Build history of the part. All positions in model axes, mm. Coordinates: 2 decimals unless noted, no trailing zeros. Order: outer loops, then holes, each group sorted by start corner. A loop starts at its lowest first (then second) coordinate and runs counter-clockwise, first axis right, second up. Notation, with made-up numbers: (26, 28) -> (44, 28) arc R25 cw to (44, 41) -> close; hole circle Ø9 at (28.5, 34). An arc over 180 degrees is marked (long way). Write each question's results on one line, items separated by ' | '.
from build123d import *

# Parameters (mm, degrees)
SKETCH1_R           = 2
BOSS_EXTRUDE1_DEPTH = 5.1


with BuildPart() as part:
    # Sketch1 → Boss-Extrude1 (new body)
    with BuildSketch(Plane.XY):
        with BuildLine():
            Line((-42.484250182, 62.101563959), (-42.484250182, 52.101563959))
            Line((-42.484250182, 52.101563959), (-57.610510686, 52.101563959))
            Line((-57.610510686, 52.101563959), (-57.610510686, 42.101563959))
            Line((-57.610510686, 42.101563959), (-2.484250182, -7.898436041))
            Line((-2.484250182, -7.898436041), (7.515749818, -7.898436041))
            Line((7.515749818, -7.898436041), (7.515749818, -17.898436041))
            Line((7.515749818, -17.898436041), (57.515749818, -17.898436041))
            Line((57.515749818, -17.898436041), (57.515749818, -7.898436041))
            Line((57.515749818, -7.898436041), (67.599923488, -7.898436041))
            Line((67.599923488, -7.898436041), (67.599923488, 2.101563959))
            Line((67.599923488, 2.101563959), (4.022842983, 38.364289155))
            ThreePointArc((4.022842983, 38.364289155), (3.080536426, 40.614131219), (5.013739676, 42.101563959))
            Line((5.013739676, 42.101563959), (22.642010323, 42.101563959))
            Line((22.642010323, 42.101563959), (22.642010323, 52.101563959))
            Line((22.642010323, 52.101563959), (7.515749818, 52.101563959))
            Line((7.515749818, 52.101563959), (7.515749818, 62.101563959))
            Line((7.515749818, 62.101563959), (-42.484250182, 62.101563959))
        make_face()
        with Locations((-32.484250182, 59.201563959)):
            Circle(SKETCH1_R, mode=Mode.SUBTRACT)
        with Locations((-2.484250182, 59.201563959)):
            Circle(SKETCH1_R, mode=Mode.SUBTRACT)
        with Locations((17.515749818, -14.998436041)):
            Circle(SKETCH1_R, mode=Mode.SUBTRACT)
        with Locations((47.515749818, -14.998436041)):
            Circle(SKETCH1_R, mode=Mode.SUBTRACT)
    extrude(amount=BOSS_EXTRUDE1_DEPTH)


solid = part.part
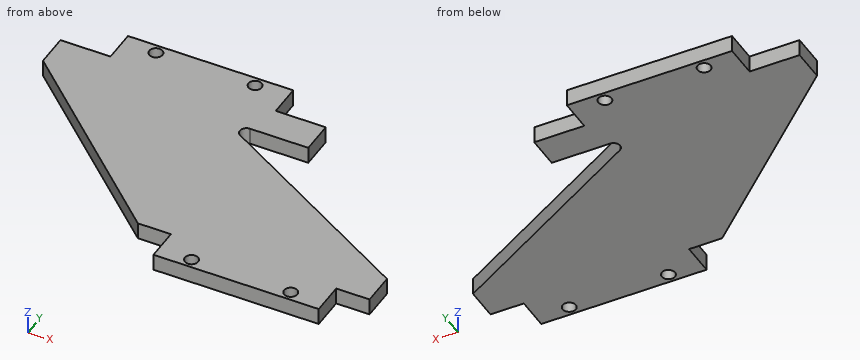
Item 1: Slice it at B-B, the plane x = -16.5. List the corners of the cut face in (y, z).
Answer:
outline: (4.81, 0) -> (62.1, 0) -> (62.1, 5.1) -> (4.81, 5.1) -> close
Item 2: Pin check, flat tips, straight feed: pin 1 (1.5 mm diameter, centred on x = 14.5, z = 1.5, fed in from +Y); pin 2 (2.5 mm diameter, centred on y = 59.5, z = 2.5, fed in from +X); pin 3 (1.5 mm diameter, centred on y = -15, z = 3.5, fed in from -X). Stop position of each tip, or through.
Answer:
pin 1: stops at y = 52.1 | pin 2: stops at x = 7.52 | pin 3: stops at x = 7.52
Item 3: Slice it at A-A, the plane z = 3.1. List the corners of the cut face in (x, y).
Answer:
outline: (-57.61, 42.1) -> (-2.48, -7.9) -> (7.52, -7.9) -> (7.52, -17.9) -> (57.52, -17.9) -> (57.52, -7.9) -> (67.6, -7.9) -> (67.6, 2.1) -> (4.02, 38.36) arc R2 cw to (5.01, 42.1) -> (22.64, 42.1) -> (22.64, 52.1) -> (7.52, 52.1) -> (7.52, 62.1) -> (-42.48, 62.1) -> (-42.48, 52.1) -> (-57.61, 52.1) -> close; hole circle Ø4 at (-32.48, 59.2); hole circle Ø4 at (-2.48, 59.2); hole circle Ø4 at (17.52, -15); hole circle Ø4 at (47.52, -15)
Item 4: Drill centre lines: line 1 (Y direction, x = -4, z = 3.95); line 2 (X direction, y = -8, z = 3.7); line 3 (Y direction, x = 62.5, z = 4.8). Where is each one in solid material? Low to high. Write a range as from..to.
Answer:
line 1: y = -6.52..57.9, 60.51..62.1 | line 2: x = 7.52..57.52 | line 3: y = -7.9..5.01
Item 5: Slice it at C-C, the plane y = 30. List the corners of the cut face in (x, z), and give its area (3 significant figures).
Answer:
outline: (-44.27, 0) -> (18.69, 0) -> (18.69, 5.1) -> (-44.27, 5.1) -> close | area: 321 mm^2
